Read the model definition and answer for the solid it produces. Units are mm, in the model's axes. A direction names the side the tool comes from. Coordinates: 2 decimals unless noted, no trailing zeros. Write each loop counter-clockwise with the first axis right and the second up, starting at its lowest first coordinate (ties: lowest second). Pieces come first, ordered by that corner, then holes. Notation, with made-up numbers: (33.5, 19) -> (90.5, 19) arc R20 ccw to (90.5, 58) -> close; hole circle Ø6 at (25.25, 61.5). An arc over 180 degrees is marked (long way). One line per item, written item: value. Start each with the question number.
1. For faces 1 (the flat face through (0, -8, -3.031)), 2 (the flat face through (0, -8, 3.031)), 3 (the flat face through (4, 2, -6)), determine the directions among +Z, -Z, +X, -X, +Y, -Y from which every point of the face is accessible in a straight line to the end or side of a thin tool.
2. Find section B-B, the plane z = -1.5. Write down the section's boundary in (x, y).
3. Find section C-C, the plane x = -5. Write down the section's boundary in (y, z).
4. Find section D-D, the plane z = 3.75. Write down the section's boundary in (x, y).
5. Consider line 1 along Y through (x, z) = (6, -0.5); line 2 along Y through (x, z) = (5.75, -3.25); line 3 along X through (y, z) = (11.25, 0). Determine where each line is inside the solid, lowest interval first.
6. Find section A-A, the plane x = 0. Write down the section's boundary in (y, z).
7. Given P1, Ø1.5, axis at x = -5.5, y = -2, coming from the -Z side; P2, Ø1.8, axis at x = -1, y = -11, coming from the +Z side; P3, Ø5, axis at x = 5.5, y = -5.5, coming from the -Z side; P4, Ø8, axis at y = 9.5, z = 0.5, coming from the -X side, each flat-ended and moving along its own axis, determine where each tip first touches the part or whether it passes through.
```python
from build123d import *

# Parameters (mm, degrees)
F0_R     = 8.75
F0_R_2   = 6.25
F1_DEPTH = 2
F2_DEPTH = 15
F3_DEPTH = 15


with BuildPart() as f1:
    # F0 (on Front) → F1 (new body)
    with BuildSketch(Plane.XZ):
        with Locations((0, -6.7e-05)):
            Circle(F0_R)
        with Locations((0, -6.7e-05)):
            Circle(F0_R_2, mode=Mode.SUBTRACT)
    extrude(amount=-F1_DEPTH)

    # F0 (on Front) → F2 (join)
    with BuildSketch(Plane.XZ):
        with Locations((0, -6.7e-05)):
            Circle(F0_R_2)
        Polygon((1.75, -3.031089), (-1.75, -3.031089), (-3.5, 0), (-1.75, 3.031089), (1.75, 3.031089), (3.5, 0), align=None, mode=Mode.SUBTRACT)
    extrude(amount=-F2_DEPTH)

    # F0 (on Front) → F3 (join, symmetric)
    with BuildSketch(Plane.XZ):
        Polygon((-3.5, 0), (-1.75, -3.031089), (1.75, -3.031089), (3.5, 0), (1.75, 3.031089), (-1.75, 3.031089), align=None)
    extrude(amount=F3_DEPTH, both=True)


solid = f1.part
```
Answer block:
1. face 1: -Z, +X, -X, -Y
1. face 2: +Z, +X, -X, -Y
1. face 3: +Y
2. outline: (-8.62, 0) -> (-2.63, 0) -> (-2.63, -15) -> (2.63, -15) -> (2.63, 0) -> (8.62, 0) -> (8.62, 2) -> (6.07, 2) -> (6.07, 15) -> (-6.07, 15) -> (-6.07, 2) -> (-8.62, 2) -> close
3. outline: (0, -7.18) -> (2, -7.18) -> (2, -3.75) -> (15, -3.75) -> (15, 3.75) -> (2, 3.75) -> (2, 7.18) -> (0, 7.18) -> close
4. outline: (-7.91, 0) -> (7.91, 0) -> (7.91, 2) -> (5, 2) -> (5, 15) -> (-5, 15) -> (-5, 2) -> (-7.91, 2) -> close
5. line 1: y = 0 to 15
5. line 2: y = 0 to 2
5. line 3: x = -6.25 to 6.25
6. outline: (-15, -3.03) -> (0, -3.03) -> (0, -8.75) -> (2, -8.75) -> (2, -6.25) -> (15, -6.25) -> (15, 6.25) -> (2, 6.25) -> (2, 8.75) -> (0, 8.75) -> (0, 3.03) -> (-15, 3.03) -> close
7. P1: passes through
7. P2: stops at z = 3.03
7. P3: stops at z = -0.87
7. P4: stops at x = -6.25
